Job drawing, mm, ordinate dimensions from the low corner. One solid piece. A direction names the side the tool comes from. Coordinates: 2 decimals unless noted, no trailing zeros. Order: outer loops, then holes, each group sorted by start corner. A loop starts at its lowest first (then second) coordinate and runs counter-clockwise, first axis right, second up. Notation, with made-up numbers: M 22,68.25 L 27,68.25 A27 cw 27,105.25 Z; hole C -4,-20.75 d8. An arc over 180 degrees is marked long. Write item = value, one per line. Start each with the question number.
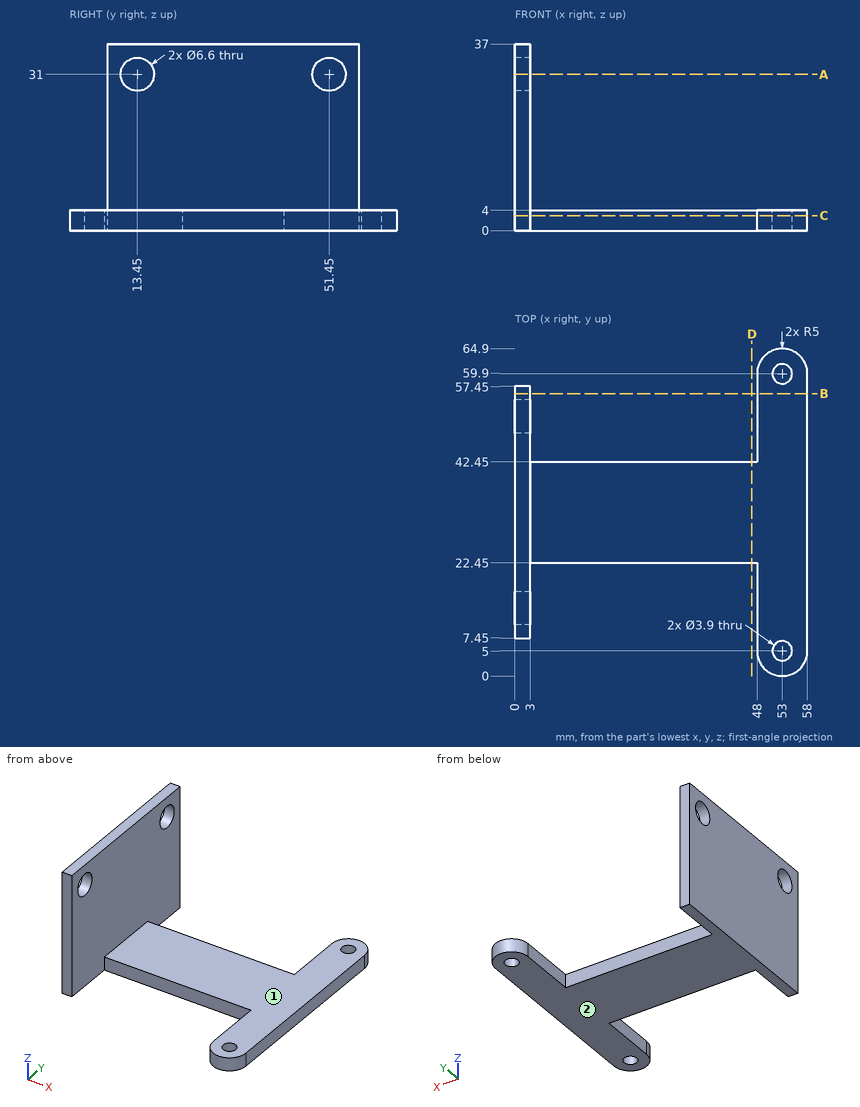
Item 1: Cut at A-A, the plane z = 31. Write the cut outline in (x, y).
Item 2: 3-axis set-ups, long thin cutter, end or side, ignore diameter. For the marked faces 1 and 2: which of +Z, -Z, +X, -X, +Y, -Y reach the whole face in a straight line?
Item 3: Cut at C-C, the plane z = 3. Write the cut outline in (x, y), and give its area (3 significant figures).
Item 4: Wall check: line 1 along Y through (x, z) = (53, 1.75); line 2 along X through (y, z) = (40.5, 28.5); line 3 along Z through (x, y) = (50, 40.5). Give the ranges that are in metal, low to high. Write a range as [from, to].
Item 5: Cut at B-B, the plane y = 56. Write the cut outline in (x, z).
Item 6: Cut at D-D, the plane x = 47. Write the cut outline in (y, z), and give its area (3 significant figures).
Item 7: Flat gauge pins, fed straight in: pin 1 (2.5 mm diameter, centred on x = 1.5, z = 17.5, fed in from +Y); pin 2 (3 mm diameter, centred on x = 17, z = 3, fed in from +Y); pin 3 (10 mm diameter, centred on y = 10.5, z = 24, fed in from +X). Where does each tip first touch, or does it go through?
Filled sheet:
q1.outline = M 0,7.45 L 3,7.45 L 3,10.15 L 0,10.15 Z; M 0,16.75 L 3,16.75 L 3,48.15 L 0,48.15 Z; M 0,54.75 L 3,54.75 L 3,57.45 L 0,57.45 Z
q2.face_1 = +Z, +X, +Y, -Y
q2.face_2 = -Z, +X, -X, +Y, -Y
q3.outline = M 0,7.45 L 3,7.45 L 3,22.45 L 48,22.45 L 48,5 A5 ccw 58,5 L 58,59.9 A5 ccw 48,59.9 L 48,42.45 L 3,42.45 L 3,57.45 L 0,57.45 Z; hole C 53,5 d3.9; hole C 53,59.9 d3.9
q3.area = 1,650 mm2
q4.line_1 = [0, 3.05], [6.95, 57.95], [61.85, 64.9]
q4.line_2 = [0, 3]
q4.line_3 = [0, 4]
q5.outline = M 0,0 L 3,0 L 3,37 L 0,37 Z; M 48,0 L 58,0 L 58,4 L 48,4 Z
q6.outline = M 22.45,0 L 42.45,0 L 42.45,4 L 22.45,4 Z
q6.area = 80.0 mm2
q7.pin_1 = 57.45
q7.pin_2 = 42.45
q7.pin_3 = 3
